Read the model definition and answer for the solid it produces. Units are mm, in the model's axes. Give positions to 0.01 mm unless a question says otherwise; leave off trailing zeros. Loops run counter-clockwise (first coordinate to the right, second up) from the corner with the lowest first, then second, coordinate; pieces in that order, holes last.
(1) Straight lines are drawn through the part: probe 1 along X at (y, z) = (0.85, -32); probe 2 along X at (y, z) = (1.9, 53); probe 3 along Z at (x, y) = (-71.5, 0.4). For each, find the intervals that lie inside material, in ascending order.
(2) Find section B-B, the plane x = -37.5. Write down the section's boundary in (y, z), then the cut area to 3 significant figures.
(3) Find section A-A, the plane z = 96.5. Write down the section's boundary in (x, y), then the cut area to 3 significant figures.
(4) Find section C-C, the plane y = 0.7. State how many separate pieces and enclosed holes the cut face has, then the cut area to 3 significant figures.
(5) This flat-tipped pin is pushed along its axis until it touches: P1, Ø3, axis at x = 96.93, z = 26, coming from the +Y side. Where does it stop, or does it pass through?
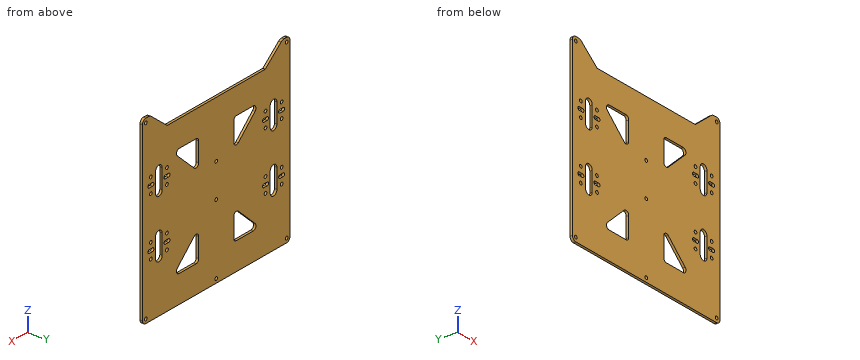
```python
from build123d import *
from build123d.topology import SkipClean

# Parameters (mm, degrees)
SKETCH1_R            = 2
BOSS_EXTRUDE2_DEPTH  = 3
FILLET1_R            = 4
FILLET1_OF_MIRROR1_R = 4


with BuildPart() as part:
    # Sketch1 → Boss-Extrude2 (new body)
    with BuildSketch(Plane(origin=(0, 0, 0), x_dir=(1, 0, 0), z_dir=(0, 1, 0))):
        with BuildLine():
            Line((-0.567360549, 109.999952103), (-0.567360549, 106.999952103))
            ThreePointArc((-0.567360549, 106.999952103), (1.432639451, 104.999952103), (-0.567360549, 102.999952103))
            Line((-0.567360549, 102.999952103), (-0.567360549, 22.499952103))
            ThreePointArc((-0.567360549, 22.499952103), (1.432639451, 20.499952103), (-0.567360549, 18.499952103))
            Line((-0.567360549, 18.499952103), (-0.567360549, -18.500047897))
            ThreePointArc((-0.567360549, -18.500047897), (1.432639451, -20.500047897), (-0.567360549, -22.500047897))
            Line((-0.567360549, -22.500047897), (-0.567360549, -89.000047897))
            Line((-0.567360549, -89.000047897), (72.593143282, -89.000047897))
            Line((72.593143282, -89.000047897), (96.205566979, -108.407802041))
            ThreePointArc((96.205566979, -108.407802041), (98.289670456, -109.589975021), (100.650361138, -110.000047897))
            Line((100.650361138, -110.000047897), (104.432639451, -110.000047897))
            ThreePointArc((104.432639451, -110.000047897), (107.968173357, -108.535581803), (109.432639451, -105.000047897))
            Line((109.432639451, -105.000047897), (109.432639451, -4.7897e-05))
            Line((109.432639451, -4.7897e-05), (109.432639451, 104.999952103))
            ThreePointArc((109.432639451, 104.999952103), (107.968173357, 108.535486009), (104.432639451, 109.999952103))
            Line((104.432639451, 109.999952103), (-0.567360549, 109.999952103))
        make_face()
        with Locations(Location((104.432639451, 104.999952103, 0), (0, 0, 90))):
            Circle(SKETCH1_R, mode=Mode.SUBTRACT)
        with Locations(Location((104.432639451, -105.000047897, 0), (0, 0, 270))):
            Circle(SKETCH1_R, mode=Mode.SUBTRACT)
        with Locations(Location((96.932639451, 25.999952103, 0), (0, 0, 90))):
            Circle(SKETCH1_R, mode=Mode.SUBTRACT)
        with Locations(Location((72.932639451, 25.999952103, 0), (0, 0, 90))):
            Circle(SKETCH1_R, mode=Mode.SUBTRACT)
        with Locations(Location((72.932639451, 43.999952103, 0), (0, 0, 90))):
            Circle(SKETCH1_R, mode=Mode.SUBTRACT)
        with Locations(Location((96.932639451, -44.000047897, 0), (0, 0, 270))):
            Circle(SKETCH1_R, mode=Mode.SUBTRACT)
        with Locations(Location((72.932639451, -44.000047897, 0), (0, 0, 270))):
            Circle(SKETCH1_R, mode=Mode.SUBTRACT)
        with Locations(Location((72.932639451, -26.000047897, 0), (0, 0, 270))):
            Circle(SKETCH1_R, mode=Mode.SUBTRACT)
        with Locations(Location((96.932639451, -26.000047897, 0), (0, 0, 270))):
            Circle(SKETCH1_R, mode=Mode.SUBTRACT)
        with Locations(Location((96.932639451, 43.999952103, 0), (0, 0, 90))):
            Circle(SKETCH1_R, mode=Mode.SUBTRACT)
        Polygon((25.578501747, 39.999952103), (25.578501747, 76.833921846), (64.808861855, 76.833921846), align=None, mode=Mode.SUBTRACT)
        Polygon((25.578501747, -20.500095793), (25.578501747, -57.061589457), (64.808861855, -57.061589457), align=None, mode=Mode.SUBTRACT)
        with BuildLine():
            Line((89.932639451, -23.164859069), (89.932639451, -46.835236724))
            ThreePointArc((89.932639451, -46.835236724), (84.932639451, -51.835236724), (79.932639451, -46.835236724))
            Line((79.932639451, -46.835236724), (79.932639451, -23.164859069))
            ThreePointArc((79.932639451, -23.164859069), (84.932639451, -18.164859069), (89.932639451, -23.164859069))
        make_face(mode=Mode.SUBTRACT)
        with BuildLine():
            Line((70.432639451, -33.000047897), (75.432639451, -33.000047897))
            ThreePointArc((75.432639451, -33.000047897), (77.432639451, -35.000047897), (75.432639451, -37.000047897))
            Line((75.432639451, -37.000047897), (70.432639451, -37.000047897))
            ThreePointArc((70.432639451, -37.000047897), (68.432639451, -35.000047897), (70.432639451, -33.000047897))
        make_face(mode=Mode.SUBTRACT)
        with BuildLine():
            Line((94.432639451, -33.000047897), (99.432639451, -33.000047897))
            ThreePointArc((99.432639451, -33.000047897), (101.432639451, -35.000047897), (99.432639451, -37.000047897))
            Line((99.432639451, -37.000047897), (94.432639451, -37.000047897))
            ThreePointArc((94.432639451, -37.000047897), (92.432639451, -35.000047897), (94.432639451, -33.000047897))
        make_face(mode=Mode.SUBTRACT)
        with BuildLine():
            Line((89.932639451, 23.164763276), (89.932639451, 46.835140931))
            ThreePointArc((89.932639451, 46.835140931), (84.932639451, 51.835140931), (79.932639451, 46.835140931))
            Line((79.932639451, 46.835140931), (79.932639451, 23.164763276))
            ThreePointArc((79.932639451, 23.164763276), (84.932639451, 18.164763276), (89.932639451, 23.164763276))
        make_face(mode=Mode.SUBTRACT)
        with BuildLine():
            Line((70.432639451, 32.999952103), (75.432639451, 32.999952103))
            ThreePointArc((75.432639451, 32.999952103), (77.432639451, 34.999952103), (75.432639451, 36.999952103))
            Line((75.432639451, 36.999952103), (70.432639451, 36.999952103))
            ThreePointArc((70.432639451, 36.999952103), (68.432639451, 34.999952103), (70.432639451, 32.999952103))
        make_face(mode=Mode.SUBTRACT)
        with BuildLine():
            Line((94.432639451, 32.999952103), (99.432639451, 32.999952103))
            ThreePointArc((99.432639451, 32.999952103), (101.432639451, 34.999952103), (99.432639451, 36.999952103))
            Line((99.432639451, 36.999952103), (94.432639451, 36.999952103))
            ThreePointArc((94.432639451, 36.999952103), (92.432639451, 34.999952103), (94.432639451, 32.999952103))
        make_face(mode=Mode.SUBTRACT)
    boss_extrude2 = extrude(amount=BOSS_EXTRUDE2_DEPTH)

    # Fillet1
    fillet1_edges = [part.edges().sort_by_distance(p)[0] for p in [
        (25.578501747, 1.5, -39.999952103),
        (64.808861855, 1.5, -76.833921846),
        (25.578501747, 1.5, -76.833921846),
        (64.808861855, 1.5, 57.061589457),
        (25.578501747, 1.5, 20.500095793),
        (25.578501747, 1.5, 57.061589457),
    ]]
    fillet(fillet1_edges, radius=FILLET1_R)

    # Mirror1: Boss-Extrude2 across plane
    with SkipClean():  # the faces are left unmerged after this step: merging them gives an invalid solid
        add(boss_extrude2.mirror(Plane(origin=(-0.567360549, 3, -102.999952103), x_dir=(0, 0, 1), z_dir=(1, 0, 0))))

    # Fillet1 of Mirror1
    fillet1_of_mirror1_edges = [part.edges().sort_by_distance(p)[0] for p in [
        (-26.713222844, 1.5, -39.999952103),
        (-65.943582953, 1.5, -76.833921846),
        (-26.713222844, 1.5, -76.833921846),
        (-65.943582953, 1.5, 57.061589457),
        (-26.713222844, 1.5, 20.500095793),
        (-26.713222844, 1.5, 57.061589457),
    ]]
    fillet(fillet1_of_mirror1_edges, radius=FILLET1_OF_MIRROR1_R)


solid = part.part
```
Entries:
1. probe 1: x = -110.57 to -91.07, -81.07 to 79.93, 89.93 to 109.43
1. probe 2: x = -110.57 to -59.78, -26.71 to 25.58, 58.65 to 109.43
1. probe 3: z = -110 to -37, -33 to 33, 37 to 89
2. outline: (0, -110) - (3, -110) - (3, -76.83) - (0, -76.83) - close; (0, -50.13) - (3, -50.13) - (3, 30.55) - (0, 30.55) - close; (0, 57.06) - (3, 57.06) - (3, 89) - (0, 89) - close
2. area: 437 mm2
3. outline: (-110.57, 0) - (-82.85, 0) - (-82.85, 3) - (-110.57, 3) - close; (81.72, 0) - (109.43, 0) - (109.43, 3) - (81.72, 3) - close
3. area: 166 mm2
4. separate pieces: 1
4. enclosed holes: 39
4. area: 40,300 mm2
5. P1: passes through
